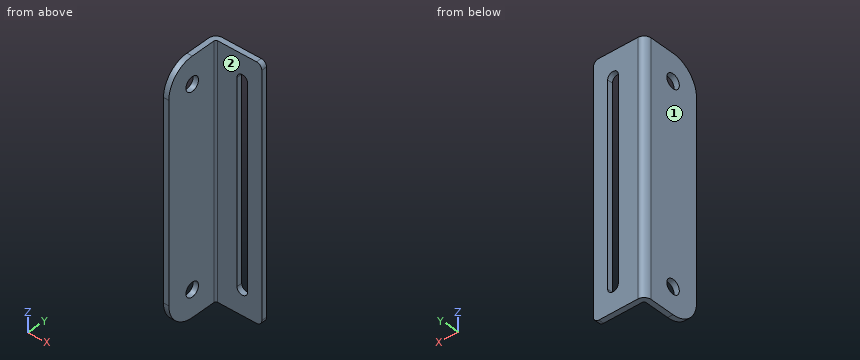
from build123d import *

# Parameters (mm, degrees)
BASE_FLANGE1_DEPTH           = 3
EDGE_FLANGE1_STRIP_W         = 14
EDGE_FLANGE1_STRIP_H         = 3
EDGE_FLANGE1_STRIP_CUT_DEPTH = 140
EDGE_FLANGE1_DEPTH           = 140
CUT_EXTRUDE1_REACH           = 84.644
SKETCH10_R                   = 4


# Sheet-metal steps are written as plain solids
with BuildPart() as part:
    # Sketch1 → Base-Flange1 (new body)
    with BuildSketch(Plane(origin=(0, 0, 0), x_dir=(1, 0, 0), z_dir=(0, 1, 0))):
        with BuildLine():
            Line((-14.5, 70), (11.5, 70))
            ThreePointArc((11.5, 70), (13.621320344, 69.121320344), (14.5, 67))
            Line((14.5, 67), (14.5, -67))
            ThreePointArc((14.5, -67), (13.621320344, -69.121320344), (11.5, -70))
            Line((11.5, -70), (-14.5, -70))
            Line((-14.5, -70), (-14.5, 70))
        make_face()
        with BuildLine():
            Line((6.5, 56), (6.5, -56))
            ThreePointArc((6.5, -56), (3.5, -59), (0.5, -56))
            Line((0.5, -56), (0.5, 56))
            ThreePointArc((0.5, 56), (3.5, 59), (6.5, 56))
        make_face(mode=Mode.SUBTRACT)
    extrude(amount=-BASE_FLANGE1_DEPTH)

    # Edge-Flange1 strip (across the edge) → Edge-Flange1 strip cut (cut)
    with BuildSketch(Plane(origin=(-14.5, -3, 70), x_dir=(1, 0, 0), z_dir=(0, 0, -1))):
        with Locations((-3, -1.5)):
            Rectangle(EDGE_FLANGE1_STRIP_W, EDGE_FLANGE1_STRIP_H)
    extrude(amount=EDGE_FLANGE1_STRIP_CUT_DEPTH, mode=Mode.SUBTRACT)

    # Edge-Flange1 section (across the edge) → Edge-Flange1 (add)
    with BuildSketch(Plane(origin=(-14.5, -3, 70), x_dir=(1, 0, 0), z_dir=(0, 0, -1))):
        with BuildLine():
            Line((0, 1), (0, 30))
            Line((0, 30), (3, 30))
            Line((3, 30), (3, 1))
            ThreePointArc((3, 1), (3.292893219, 0.292893219), (4, 0))
            Line((4, 0), (4, -3))
            ThreePointArc((4, -3), (1.171572875, -1.828427125), (0, 1))
        make_face()
    extrude(amount=EDGE_FLANGE1_DEPTH)

    # Sketch10 → Cut-Extrude1 (cut, up to next)
    with BuildSketch(Plane.ZY.offset(14.5), mode=Mode.PRIVATE) as cut_extrude1_sk1:
        with BuildLine():
            ThreePointArc((-55, -33), (-65.606601718, -28.606601718), (-70, -18))
            Line((-70, -18), (-70, -33))
            Line((-70, -33), (-55, -33))
        make_face()
    cut_extrude1_tool1 = extrude(cut_extrude1_sk1.sketch, amount=-CUT_EXTRUDE1_REACH, mode=Mode.PRIVATE) & part.part
    # Sketch10 → Cut-Extrude1 (cut, up to next)
    with BuildSketch(Plane.ZY.offset(14.5), mode=Mode.PRIVATE) as cut_extrude1_sk2:
        with BuildLine():
            Line((55, -33), (70, -33))
            Line((70, -33), (70, -18))
            ThreePointArc((70, -18), (65.606601718, -28.606601718), (55, -33))
        make_face()
    cut_extrude1_tool2 = extrude(cut_extrude1_sk2.sketch, amount=-CUT_EXTRUDE1_REACH, mode=Mode.PRIVATE) & part.part
    # Sketch10 → Cut-Extrude1 (cut, up to next)
    with BuildSketch(Plane.ZY.offset(14.5), mode=Mode.PRIVATE) as cut_extrude1_sk3:
        with Locations(Location((-55, -18, 0), (0, 0, 270))):
            Circle(SKETCH10_R)
    cut_extrude1_tool3 = extrude(cut_extrude1_sk3.sketch, amount=-CUT_EXTRUDE1_REACH, mode=Mode.PRIVATE) & part.part
    # Sketch10 → Cut-Extrude1 (cut, up to next)
    with BuildSketch(Plane.ZY.offset(14.5), mode=Mode.PRIVATE) as cut_extrude1_sk4:
        with Locations(Location((55, -18, 0), (0, 0, 270))):
            Circle(SKETCH10_R)
    cut_extrude1_tool4 = extrude(cut_extrude1_sk4.sketch, amount=-CUT_EXTRUDE1_REACH, mode=Mode.PRIVATE) & part.part
    add(cut_extrude1_tool1.solids().sort_by_distance((-14.5, -29.649481, -66.649481))[0], mode=Mode.SUBTRACT)
    add(cut_extrude1_tool2.solids().sort_by_distance((-14.5, -29.649481, 66.649481))[0], mode=Mode.SUBTRACT)
    add(cut_extrude1_tool3.solids().sort_by_distance((-14.5, -18, -55))[0], mode=Mode.SUBTRACT)
    add(cut_extrude1_tool4.solids().sort_by_distance((-14.5, -18, 55))[0], mode=Mode.SUBTRACT)


solid = part.part
Could you check a few things on this model? Use its own coordinates, in mm. Face numbers are marked on the shaded views. A direction names the side the tool comes from. Coordinates: 2 decimals unless noted, no trailing zeros. Loops run counter-clockwise (first coordinate to the right, second up) from the corner with the lowest first, then second, coordinate; pieces in that order, holes last.
1. Imagine slicing it at A-A (z = -49.5). Please give me the cut outline in (x, y).
2. Imagine slicing it at C-C (y = -11.5). Please give me the cut outline in (x, z), and give its area (3 significant figures).
3. Imagine slicing it at B-B (x = 3.5). Please give me the cut outline in (y, z), and give its area (3 significant figures).
4. For P1, Ø0.9, axis at y = -2, z = 26, coming from the -X side; P2, Ø12, axis at x = 2, z = -4, coming from the -Y side; P3, Ø9, axis at y = -18, z = -55, coming from the +X side; P4, Ø4, axis at x = 6.5, y = -5.5, coming from the -Z side, each with a flat end and sliding along its axis, tell me the tip position at first contact or that it passes through.
5. Imagine slicing it at D-D (x = 9.25). Please give me the cut outline in (y, z), and give its area (3 significant figures).
6. I need wall thicknesses on L1, parallel to Z at x = -13.35, y = -18; L2, parallel to X at y = -27.5, z = 3.5; L3, parallel to Y at x = -1.75, z = -45.5. Which ranges of each line are inside material? Lowest first, please.
7. For the marked faces 1 and 2, which set-ups out of +Z, -Z, +X, -X, +Y, -Y let a thin tool reach every point of the face, with its end or its side?
Computed values:
1. outline: (-14.5, -33) - (-11.5, -33) - (-11.5, -4) arc R1 cw to (-10.5, -3) - (0.5, -3) - (0.5, 0) - (-10.5, 0) arc R4 ccw to (-14.5, -4) - close; (6.5, -3) - (14.5, -3) - (14.5, 0) - (6.5, 0) - close
2. outline: (-14.5, -70) - (-11.5, -70) - (-11.5, 70) - (-14.5, 70) - close
2. area: 420 mm2
3. outline: (-3, -70) - (0, -70) - (0, -59) - (-3, -59) - close; (-3, 59) - (0, 59) - (0, 70) - (-3, 70) - close
3. area: 66.0 mm2
4. P1: stops at x = -14.19
4. P2: stops at y = -3
4. P3: stops at x = -11.5
4. P4: passes through
5. outline: (-3, -70) - (0, -70) - (0, 70) - (-3, 70) - close
5. area: 420 mm2
6. L1: z = -70 to -59, -51 to 51, 59 to 70
6. L2: x = -14.5 to -11.5
6. L3: y = -3 to 0
7. face 1: +Z, -Z, -X, +Y, -Y
7. face 2: +Z, -Z, +X, -Y
